For this review, use the dimensioned drawing (mm, ordinates from the lowest corner) and the shaded views. A direction names the side the tool comes from. Give positions to 0.01 mm unless a question says otherwise; leave off trailing zeros. Write each loop counter-clockwise with the first axis right and the second up, starting at its lowest first coordinate (ties: lowest second). Pieces come first, ordered by that corner, then holes. Notation, with made-up numbers: (47, 61) -> (91, 61) arc R21 cw to (91, 89) -> close; hole circle Ø11 at (44.25, 65). An arc over 180 degrees is marked (long way). Write each question's results on one line, items separated by ' | '. Start each with the question number.
(1) Take a section at A-A (x = 738). State the section outline as (y, z) points, plus the area to 3 significant figures.
(2) For the marked faces 1, 2, 3, 4 and 5, list the 3-axis set-ups (+Z, -Z, +X, -X, +Y, -Y) from which the entire face can be reached by the end or side of a thin tool; tool diameter is ignored.
(3) Clearance check with flat-ended pins moving along their axes: pin 1 (2 mm diameter, centred on y = 403.5, z = 276.5, fed in from +X); pin 2 (3 mm diameter, centred on y = 180, z = 111.5, fed in from -X); pin 3 (5 mm diameter, centred on x = 462, z = 220, fed in from +Y). State where each tip first meets the part, or that it passes through.
(4) To check wall thickness, follow probe 1 along X at (y, z) = (462, 75); probe 2 along Y at (x, z) = (520, 278.5); probe 3 along Z at (x, y) = (929.5, 443.5). State the ranges of each line that lie inside material, in increasing order.
(5) Take a section at B-B (y = 804). State the section outline as (x, z) points.
(6) Take a section at D-D (y = 937). State the section outline as (x, z) points, plus the area to 3 significant figures.
(7) Take a section at C-C (z = 275). State the section outline as (x, y) points, plus the area to 3 significant figures.
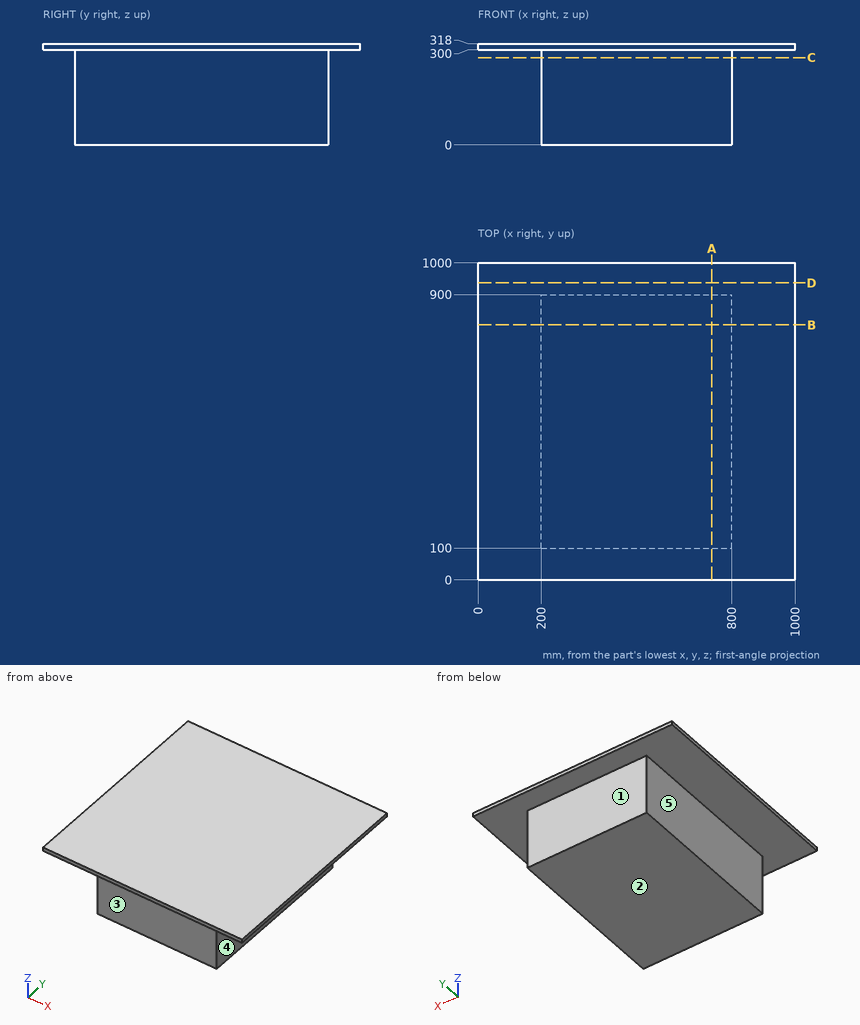
Report:
1) outline: (0, 300) -> (100, 300) -> (100, 0) -> (900, 0) -> (900, 300) -> (1000, 300) -> (1000, 318) -> (0, 318) -> close | area: 258,000 mm2
2) face 1: -Z, +X, -X, +Y | face 2: -Z, +X, -X, +Y, -Y | face 3: -Z, +X, -X, -Y | face 4: -Z, +X, +Y, -Y | face 5: -Z, -X, +Y, -Y
3) pin 1: x = 800 | pin 2: x = 200 | pin 3: y = 900
4) probe 1: 200 to 800 | probe 2: 100 to 900 | probe 3: 300 to 318
5) outline: (0, 300) -> (200, 300) -> (200, 0) -> (800, 0) -> (800, 300) -> (1000, 300) -> (1000, 318) -> (0, 318) -> close
6) outline: (0, 300) -> (1000, 300) -> (1000, 318) -> (0, 318) -> close | area: 18,000 mm2
7) outline: (200, 100) -> (800, 100) -> (800, 900) -> (200, 900) -> close | area: 480,000 mm2
